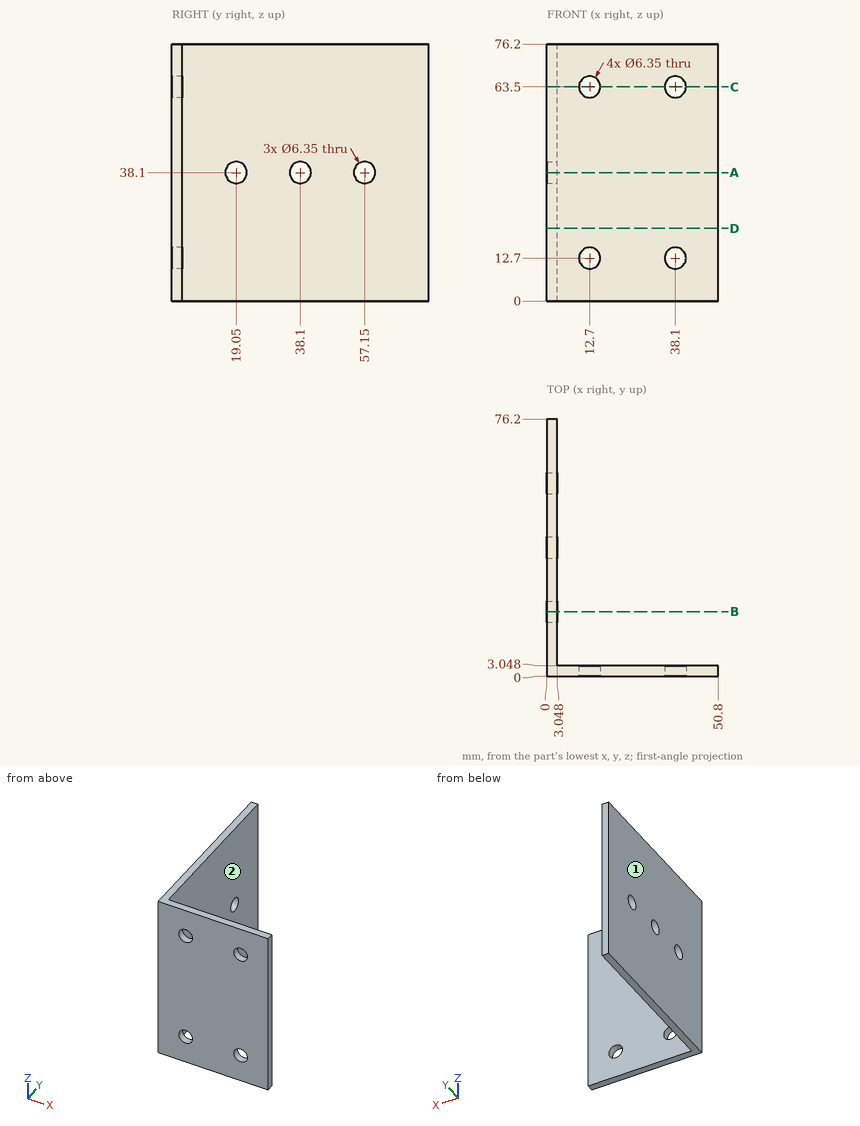
Part print with two shaded views. Sizes in mm from the minimum x, y, z corner. A direction names the side the tool comes from. Coordinates: 2 decimals unless noted, no trailing zeros. Write each loop counter-clockwise with the first axis right and the second up, starting at its lowest first coordinate (ties: lowest second). Pieces come first, ordered by that corner, then holes. Notation, with made-up numbers: (-37.5, 74.5) - (17.5, 74.5) arc R36 ccw to (17.5, 108.5) - close; hole circle Ø11 at (70.5, 81.25). An arc over 180 degrees is marked (long way). Put each result on its own line as item: value.
1. Band-saw the part on C-C (z = 63.5). Write the cut outline in (x, y) (3 decimals).
Final values:
outline: (0, 0) - (9.525, 0) - (9.525, 3.048) - (3.048, 3.048) - (3.048, 76.2) - (0, 76.2) - close; (15.875, 0) - (34.925, 0) - (34.925, 3.048) - (15.875, 3.048) - close; (41.275, 0) - (50.8, 0) - (50.8, 3.048) - (41.275, 3.048) - close
2. 3-axis set-ups, long thin cutter, end or side, ignore diameter. For the marked faces 1 and 2: which of +Z, -Z, +X, -X, +Y, -Y reach the whole face in a straight line?
Final values:
face 1: +Z, -Z, -X, +Y, -Y
face 2: +Z, -Z, +X, +Y
3. Band-saw the part on A-A (z = 38.1). Write the cut outline in (x, y) (3 decimals).
Final values:
outline: (0, 0) - (50.8, 0) - (50.8, 3.048) - (3.048, 3.048) - (3.048, 15.875) - (0, 15.875) - close; (0, 22.225) - (3.048, 22.225) - (3.048, 34.925) - (0, 34.925) - close; (0, 41.275) - (3.048, 41.275) - (3.048, 53.975) - (0, 53.975) - close; (0, 60.325) - (3.048, 60.325) - (3.048, 76.2) - (0, 76.2) - close
4. Band-saw the part on B-B (y = 19.05). Write the cut outline in (x, z) (3 decimals), then the cut area to 3 significant figures.
Final values:
outline: (0, 0) - (3.048, 0) - (3.048, 34.925) - (0, 34.925) - close; (0, 41.275) - (3.048, 41.275) - (3.048, 76.2) - (0, 76.2) - close
area: 213 mm²
5. Flat gauge pins, fed straight in: pin 1 Ø14.5 at (x, z) = (25.5, 39.5) entering from +Y; pin 2 Ø8 at (y, z) = (49, 28.5) entering from +X. Where does each tip first touch, or does it go through?
Final values:
pin 1: stops at y = 3.05
pin 2: stops at x = 3.05
6. Band-saw the part on D-D (z = 21.5). Write the cut outline in (x, y), then the cut area to 3 significant figures.
Final values:
outline: (0, 0) - (50.8, 0) - (50.8, 3.05) - (3.05, 3.05) - (3.05, 76.2) - (0, 76.2) - close
area: 378 mm²
7. Probe line 1 along Z through (x, y) = (2, 38); line 2 along X through (y, z) = (1.2, 63.5) (3 decimals); line 3 along X through (y, z) = (1, 12). List the from-to ranges inside material, lowest first. Write a range as [from, to].
Final values:
line 1: z = [0, 34.93], [41.27, 76.2]
line 2: x = [0, 9.525], [15.875, 34.925], [41.275, 50.8]
line 3: x = [0, 9.6], [15.8, 35], [41.2, 50.8]
